Check sheet for the modelled part. Datum: model origin and axes. Units: mm. Face numbers are marked on the shaded views. A direction names the side the tool comes from. Round coordinates to 2 decimals unless told otherwise and drop trailing zeros. Order: outer loops, then holes, each group sorted by start corner. A loop starts at its lowest first (then second) coordinate and runs counter-clockwise, first axis right, second up. Notation, with made-up numbers: (14, 15.25) -> (23, 15.25) arc R35 cw to (23, 53.25) -> close; hole circle Ø3 at (43, 81). An arc over 180 degrees is marked (long way). Answer in a Markdown table with one row per item.
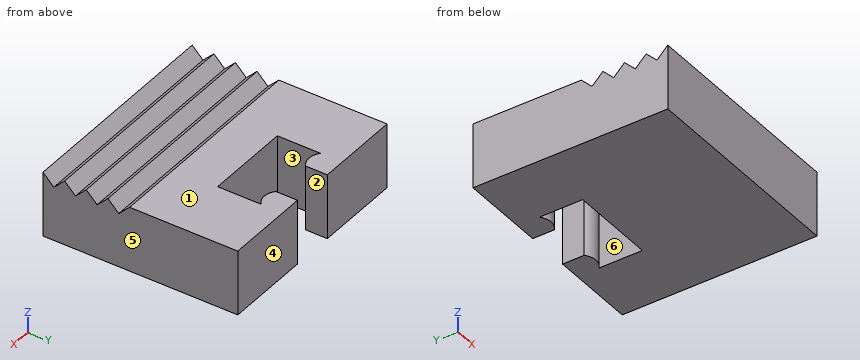
Autodesk Inventor part; units mm, degrees
ref_plane "YZ Plane" through (0, 0, 0) normal (1, 0, 0) x (0, 1, 0)
ref_plane "XZ Plane" through (0, 0, 0) normal (0, 1, 0) x (-1, 0, 0)
ref_plane "XY Plane" through (0, 0, 0) normal (0, 0, 1) x (1, 0, 0)
sketch "Sketch1" plane through (0, 0, 0) normal (0, 0, 1) x (1, 0, 0)
  line L0 (0, 0) -> (10, 0)
  line L1 (10, 0) -> (10, 9)
  line L2 (10, 9) -> (0, 9)
  line L3 (0, 9) -> (0, 0)
  point P0 (5, 9)
  dimension "d0" = 10
  dimension "d1" = 9
extrude "Extrusion1" add sketch "Sketch1" along normal blind 3
sketch "Sketch10" plane through (0, 0, 0) normal (-1, 0, 0) x (0, 0, 1)
  line L0 (0, 0) -> (3, 0)
  line L1 (3, 0) -> (2.5, 0)
  line L2 (2.5, 0) -> (2.5, 0.5)
  line L3 (2.5, 6) -> (3, 6)
  line L4 (3, 6) -> (3, 4)
  line L5 (3, 0) -> (3.7071, 0) construction
  line L6 (2.5, 4.25) -> (3, 4.25)
  line L7 (3, 1) -> (2.5, 1.5)
  line L8 (2.5, 1.5) -> (3, 2)
  line L9 (3, 2) -> (2.5, 2.5)
  line L10 (2.5, 2.5) -> (3, 3)
  line L11 (3, 3) -> (2.5, 3.5)
  line L12 (2.5, 3.5) -> (3, 4)
  line L13 (3, 4) -> (3, 4.25)
  line L14 (3, 1) -> (3, 0)
  line L15 (3, 2) -> (3, 1)
  line L16 (3, 4) -> (3, 3)
  line L17 (2.5, 2.5) -> (2.5, 3.5)
  line L18 (2.5, 1.5) -> (2.5, 2.5)
  line L19 (2.5, 0.5) -> (2.5, 1.5)
  line L20 (2.5, 3.5) -> (2.5, 6)
  line L21 (3, 3) -> (3, 2)
  line L22 (3, 1) -> (2.5, 0.5)
  line L23 (2.5, 0.5) -> (3, 0)
  point P0 (2.5, 3)
  dimension "d23" = 0.5
  dimension "d24" = 6
sketch "Sketch12" plane through (0, 0, 3) normal (0, 0, 1) x (1, 0, 0)
  line L0 (10, 9) -> (0, 9)
  line L1 (7, 6) -> (3, 6)
  line L2 (3, 6) -> (3, 8)
  line L3 (3, 8) -> (7, 8)
  line L4 (7, 8) -> (7, 6)
  line L5 (7, 6) -> (3, 8) construction
  line L6 (3, 6) -> (7, 8) construction
  line L7 (6, 7) -> (4, 7)
  line L8 (4, 7) -> (4, 9)
  line L9 (4, 9) -> (6, 9)
  line L10 (6, 9) -> (6, 7)
  line L11 (6, 7) -> (4, 9) construction
  line L12 (4, 7) -> (6, 9) construction
  line L13 (0, 9) -> (0, 0)
  point P0 (5, 7)
  point P1 (5, 8)
  dimension "d47" = 2
  dimension "d48" = 4
  dimension "d49" = 2
  dimension "d50" = 2
  dimension "d68" = 5
extrude "Extrusion10" cut sketch "Sketch12" against normal up to next
extrude "Extrusion13" cut sketch "Sketch10" against normal up to next contours L23 L22 L14 | L7 L8 L15 | L9 L10 L21 | L11 L12 L16
sketch "Sketch16" plane through (0, 0, 0) normal (0, 0, -1) x (-1, 0, 0)
  line L0 (-7, 8) -> (-6, 8)
  arc A0 (-7, 8) -> (-6, 8) centre (-6.5, 8.559) ccw
  line L1 (-4, 8) -> (-3, 8)
  line L2 (-3, 8) -> (-3, 6)
  arc A1 (-4, 8) -> (-3, 8) centre (-3.5, 8.559) ccw
  point P0 (0, 0)
  dimension "d69" = 0.75
  dimension "d70" = 0.75
extrude "Extrusion14" add sketch "Sketch16" against normal up to surface (3 mm away)
properties part number "Clamp-part2(moving)-Base9x10mm."
(1) Section check B-B on z = 1.9. Record the boundary of the cut face in (x, y).
Solutions:
| item | result |
|---|---|
| outline | (0, 0) -> (10, 0) -> (10, 9) -> (6, 9) -> (6, 8) arc R0.75 ccw to (7, 8) -> (7, 6) -> (3, 6) -> (3, 8) arc R0.75 ccw to (4, 8) -> (4, 9) -> (0, 9) -> close |
(2) Tool access check on the marked faces 1, 2 and 3. Record the directions out of +Z, -Z, +X, -X, +Y, -Y that give a thin tool (end or side, any length) a straight path to the whole face; none if there is none.
Solutions:
| item | result |
|---|---|
| face 1 | +Z, +X, -X, +Y, -Y |
| face 2 | +Z, -Z, +Y |
| face 3 | +Z, -Z |
(3) Scan lines: probe 1 along X at (y, z) = (7, 2.2); probe 2 along Y at (x, z) = (3.5, 0.3); probe 3 along Y at (x, z) = (4.75, 1.05). Record each from-to range of solid material in increasing order. Write a range as from..to.
Solutions:
| item | result |
|---|---|
| probe 1 | 0..3, 7..10 |
| probe 2 | 0..6, 7.81..9 |
| probe 3 | 0..6 |
(4) Draft check along X on the marked faces 4, 5 and 6. Enter one of: pulls with the +X half, pulls with the -X half, needs draft (parallel to the pull), parting line crosses it, or undercut.
Solutions:
| item | result |
|---|---|
| face 4 | needs draft |
| face 5 | pulls with the +X half |
| face 6 | undercut |
(5) Section check C-C on x = 8. Record the boundary of the cut face in (y, z), plus the area to 3 significant figures.
Solutions:
| item | result |
|---|---|
| outline | (0, 0) -> (9, 0) -> (9, 3) -> (4, 3) -> (3.5, 2.5) -> (3, 3) -> (2.5, 2.5) -> (2, 3) -> (1.5, 2.5) -> (1, 3) -> (0.5, 2.5) -> (0, 3) -> close |
| area | 26.0 mm^2 |
(6) Section check D-D on y = 2.75. Record the boundary of the cut face in (x, z).
Solutions:
| item | result |
|---|---|
| outline | (0, 0) -> (10, 0) -> (10, 2.75) -> (0, 2.75) -> close |
(7) Section check A-A on y = 7.25. Record the boundary of the cut face in (x, z), plus the area to 3 significant figures.
Solutions:
| item | result |
|---|---|
| outline | (0, 0) -> (3, 0) -> (3, 3) -> (0, 3) -> close; (7, 0) -> (10, 0) -> (10, 3) -> (7, 3) -> close |
| area | 18.0 mm^2 |
